from build123d import *

# Parameters (mm, degrees)
SKETCH_1_W          = 100
SKETCH_1_H          = 100
EXTRUDE_1_DEPTH     = 10
SKETCH_2_R          = 5
CUT_EXTRUDE_1_DEPTH = 10
SKETCH_3_R          = 5
CUT_EXTRUDE_2_DEPTH = 10
SKETCH_4_R          = 5
CUT_EXTRUDE_3_DEPTH = 10


with BuildPart() as part:
    # Эскиз1 → Бобышка-Вытянуть1 (new body)
    with BuildSketch(Plane.XY):
        with Locations((50, 50)):
            Rectangle(SKETCH_1_W, SKETCH_1_H)
    extrude(amount=EXTRUDE_1_DEPTH)

    # Эскиз2 → Вырез-Вытянуть1 (cut)
    with BuildSketch(Plane.XY):
        with Locations((0, 3)):
            Circle(SKETCH_2_R)
    extrude(amount=CUT_EXTRUDE_1_DEPTH, mode=Mode.SUBTRACT)

    # Эскиз3 → Вырез-Вытянуть2 (cut)
    with BuildSketch(Plane.XY):
        with Locations((1.2, 33.6)):
            Circle(SKETCH_3_R)
    extrude(amount=CUT_EXTRUDE_2_DEPTH, mode=Mode.SUBTRACT)

    # Эскиз4 → Вырез-Вытянуть3 (cut)
    with BuildSketch(Plane.XY):
        with Locations((8.5, 99)):
            Circle(SKETCH_4_R)
    extrude(amount=CUT_EXTRUDE_3_DEPTH, mode=Mode.SUBTRACT)


solid = part.part
Check sheet for the modelled part. Datum: model origin and axes. Units: mm. Coordinates: 2 decimals unless noted, no trailing zeros. Loops run counter-clockwise (first coordinate to the right, second up) from the corner with the lowest first, then second, coordinate; pieces in that order, holes last. Notation, with made-up numbers: (81.5, 2.5) -> (89.5, 2.5) arc R18 ccw to (89.5, 25.5) -> close; hole circle Ø8 at (-27.5, 22). An arc over 180 degrees is marked (long way). Answer in a Markdown table with one row per item.
1. Sectioned sample at A-A, the plane x = 1.2. Record the boundary of the cut face in (y, z), then the cut area to 3 significant figures.
Check values:
| item | result |
|---|---|
| outline | (7.85, 0) -> (28.6, 0) -> (28.6, 10) -> (7.85, 10) -> close; (38.6, 0) -> (100, 0) -> (100, 10) -> (38.6, 10) -> close |
| area | 821 mm2 |
2. Go/stop test with a flat-tipped pin: pin 1 (9 mm diameter, centred on x = 1.2, y = 33.6, fed in from +Z). Record where the tip stops, or that it passes through.
Check values:
| item | result |
|---|---|
| pin 1 | passes through |
3. Sectioned sample at B-B, the plane y = 33.6. Record the boundary of the cut face in (x, z), then the cut area to 3 significant figures.
Check values:
| item | result |
|---|---|
| outline | (6.2, 0) -> (100, 0) -> (100, 10) -> (6.2, 10) -> close |
| area | 938 mm2 |
4. Material ranges on line 1 along X through (y, z) = (33.6, 2.5); line 2 along Y through (x, z) = (8.5, 7.25); line 3 along X through (y, z) = (38, 6), recorded low to high. Write a range as [from, to].
Check values:
| item | result |
|---|---|
| line 1 | x = [6.2, 100] |
| line 2 | y = [0, 94] |
| line 3 | x = [3.57, 100] |
5. Release check for a two-part mould opening along X. For faces 1 (the face through (100, 49, 5)), 2 (the face through (0, 69, 5)), 3 (the face through (51, 0, 5)), 4 (the face through (8.4, 94, 4.9)) record: released by +X, released by -X, zero draft, split by the parting line, or undercut.
Check values:
| item | result |
|---|---|
| face 1 | released by +X |
| face 2 | released by -X |
| face 3 | zero draft |
| face 4 | undercut |
